The listing builds one solid part. Answer for the finished solid, in the listing's coordinates (mm). Round coordinates to 2 decimals unless told otherwise and drop trailing zeros. Order: outer loops, then holes, each group sorted by start corner. A loop starts at its lowest first (then second) coordinate and runs counter-clockwise, first axis right, second up. Notation, with made-up numbers: (-3.5, 64.5) - (26.5, 64.5) arc R17 ccw to (26.5, 79.5) - close; hole circle Ø7 at (16, 80). An arc over 180 degrees is marked (long way). Write item = value, one per line.
from build123d import *

# Parameters (mm, degrees)
CROQUIS1_W              = 416
CROQUIS1_H              = 96
CROQUIS1_W_2            = 384
CROQUIS1_H_2            = 64
CROQUIS1_W_3            = 20.00615983
CROQUIS1_H_3            = 6
SALIENTE_EXTRUIR1_DEPTH = 3


with BuildPart() as part:
    # Croquis1 → Saliente-Extruir1 (new body)
    with BuildSketch(Plane(origin=(0, 0, 0), x_dir=(1, 0, 0), z_dir=(0, 1, 0))):
        Rectangle(CROQUIS1_W, CROQUIS1_H)
        Rectangle(CROQUIS1_W_2, CROQUIS1_H_2, mode=Mode.SUBTRACT)
        with Locations((197.996920085, -51)):
            Rectangle(CROQUIS1_W_3, CROQUIS1_H_3)
        with Locations((197.996920085, 51)):
            Rectangle(CROQUIS1_W_3, CROQUIS1_H_3)
        with Locations((-197.996920085, 51)):
            Rectangle(CROQUIS1_W_3, CROQUIS1_H_3)
        with Locations((-197.996920085, -51)):
            Rectangle(CROQUIS1_W_3, CROQUIS1_H_3)
    extrude(amount=SALIENTE_EXTRUIR1_DEPTH)


solid = part.part
Q1. Find the intervals of material crossed by line 1 (Z direction, x = 39.5, y = 0.2); line 2 (X direction, y = 1.45, z = 23); line 3 (X direction, y = 2.6, z = 49.5), in increasing order. Write a range as from..to.
Model answer:
line_1 = -48..-32, 32..48
line_2 = -208..-192, 192..208
line_3 = -208..-187.99, 187.99..208
Q2. Section B-B on y = 1.85 is taken. Determine the outline of the cut face in (x, z).
Model answer:
outline = (-208, -54) - (-187.99, -54) - (-187.99, -48) - (187.99, -48) - (187.99, -54) - (208, -54) - (208, 54) - (187.99, 54) - (187.99, 48) - (-187.99, 48) - (-187.99, 54) - (-208, 54) - close; hole (-192, -32) - (192, -32) - (192, 32) - (-192, 32) - close
Q3. Section A-A on x = 148.5 is taken. Determine the outline of the cut face in (y, z).
Model answer:
outline = (0, -48) - (3, -48) - (3, -32) - (0, -32) - close; (0, 32) - (3, 32) - (3, 48) - (0, 48) - close
Q4. Flat-ended cylindrical pins translate along their axes: P1, Ø0.9, axis at x = 69, y = 1, coming from the +Z side; P2, Ø0.9, axis at x = 80, y = 1.5, coming from the -Z side. Find the tip coordinate at first contact, or state that the pin passes through.
Model answer:
P1 = 48
P2 = -48
Q5. Section C-C on z = -11 is taken. Determine the outline of the cut face in (x, y), then the cut area to 3 significant figures.
Model answer:
outline = (-208, 0) - (-192, 0) - (-192, 3) - (-208, 3) - close; (192, 0) - (208, 0) - (208, 3) - (192, 3) - close
area = 96.0 mm^2
